Check sheet for the modelled part. Datum: model origin and axes. Units: mm. Face numbers are marked on the shaded views. A direction names the side the tool comes from. Round coordinates to 2 decimals unless told otherwise and drop trailing zeros. Write each loop counter-clockwise with the first axis right and the second up, starting at its lowest first coordinate (ties: lowest second). Pieces come first, ordered by that corner, then holes. Notation, with made-up numbers: (87.5, -7) - (127.5, -7) arc R27 ccw to (127.5, 9) - close; hole circle Ø7 at (-18.5, -38.75). An arc over 180 degrees is marked (long way). Use one line per item in the form item = value. Start each with the question number.
1) Section check B-B (y = -2.5). Record the boundary of the cut face in (x, z), then the cut area to 4 significant figures.
2) Section check C-C (x = -1.3). Record the boundary of the cut face in (y, z).
3) Gauge pin test, flat ends, axial feed: P1, Ø1, axis at x = 0, y = -1, coming from the -Z side; P2, Ø2.5, axis at x = 1, z = 32, coming from the -Y side; P3, Ø1.7, axis at x = 0, y = -2.5, coming from the +Z side. Record the tip position at first contact, or that the pin passes through.
4) Set-up check for the marked faces 1, 2 and 3: record each of +Z, -Z, +X, -X, +Y, -Y from which the full face is reachable in a straight line by a thin tool's end or side.
5) Section check A-A (z = 23.5). Record the boundary of the cut face in (x, y).
6) Scan lines: probe 1 along Z at (x, y) = (0.7, -2.5); probe 2 along Z at (x, y) = (-1.3, -3); probe 3 along Y at (x, z) = (0.15, 8). Record each from-to range of solid material in increasing order.
7) Section check D-D (z = 28.5). Record the boundary of the cut face in (x, y).
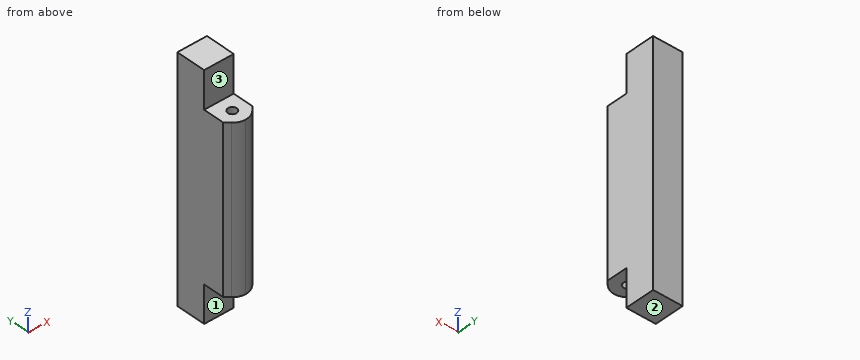
from build123d import *

# Parameters (mm, degrees)
SKETCH_1_W          = 5
SKETCH_1_H          = 10
EXTRUDE_1_DEPTH     = 27.5
SKETCH_2_W          = 5
SKETCH_2_H          = 5
EXTRUDE_2_DEPTH     = 20
SKETCH_3_R          = 0.75
CUT_EXTRUDE_1_DEPTH = 6
CUT_EXTRUDE_2_DEPTH = 27.5


with BuildPart() as part:
    # 草图1 → 凸台-拉伸1 (new body)
    with BuildSketch(Plane.XY):
        Rectangle(SKETCH_1_W, SKETCH_1_H)
    extrude(amount=EXTRUDE_1_DEPTH)

    # 草图2 → 凸台-拉伸2 (add, symmetric)
    with BuildSketch(Plane.XY.offset(13.75)):
        with Locations((0, 2.5)):
            Rectangle(SKETCH_2_W, SKETCH_2_H)
    extrude(amount=EXTRUDE_2_DEPTH, both=True)

    # 草图3 → 切除-拉伸1 (cut)
    with BuildSketch(Plane(origin=(0, 0, 0), x_dir=(-1, 0, 0), z_dir=(0, 0, -1))):
        with Locations((0, -2.5)):
            Circle(SKETCH_3_R)
    cut_extrude_1 = extrude(amount=-CUT_EXTRUDE_1_DEPTH, mode=Mode.SUBTRACT)

    # 镜向1: 切除-拉伸1 across plane
    add(cut_extrude_1.mirror(Plane.XY.offset(13.75)), mode=Mode.SUBTRACT)

    # 草图4 → 切除-拉伸2 (cut)
    with BuildSketch(Plane(origin=(0, 0, 0), x_dir=(-1, 0, 0), z_dir=(0, 0, -1))):
        with BuildLine():
            ThreePointArc((0, -5), (-0.956708581, -4.809698831), (-1.767766953, -4.267766953))
            Line((-1.767766953, -4.267766953), (-2.5, -3.535533906))
            Line((-2.5, -3.535533906), (-2.5, -5))
            Line((-2.5, -5), (0, -5))
        make_face()
        with BuildLine():
            ThreePointArc((1.767766953, -4.267766953), (0.956708581, -4.809698831), (0, -5))
            Line((0, -5), (2.5, -5))
            Line((2.5, -5), (2.5, -3.535533906))
            Line((2.5, -3.535533906), (1.767766953, -4.267766953))
        make_face()
    extrude(amount=-CUT_EXTRUDE_2_DEPTH, mode=Mode.SUBTRACT)


solid = part.part
Results are:
q1.outline = (-2.5, 0) - (-0.75, 0) - (-0.75, 6) - (0.75, 6) - (0.75, 0) - (2.5, 0) - (2.5, 27.5) - (0.75, 27.5) - (0.75, 21.5) - (-0.75, 21.5) - (-0.75, 27.5) - (-2.5, 27.5) - close
q1.area = 119.5 mm²
q2.outline = (-4.64, 0) - (0, 0) - (0, -6.25) - (5, -6.25) - (5, 33.75) - (0, 33.75) - (0, 27.5) - (-4.64, 27.5) - close
q3.P1 = 0
q3.P2 = 0
q3.P3 = 27.5
q4.face_1 = -Z, +X, -X, -Y
q4.face_2 = -Z, +X, -X, +Y, -Y
q4.face_3 = +Z, +X, -X, -Y
q5.outline = (-2.5, -3.54) - (-1.77, -4.27) arc R2.5 ccw to (1.77, -4.27) - (2.5, -3.54) - (2.5, 5) - (-2.5, 5) - close; hole circle Ø1.5 at (0, -2.5)
q6.probe_1 = 6 to 21.5
q6.probe_2 = 0 to 27.5
q6.probe_3 = -5 to 5
q7.outline = (-2.5, 0) - (2.5, 0) - (2.5, 5) - (-2.5, 5) - close
